Geometry: final body of the model. Coordinates: model frame, mm. Face numbers are marked on the shaded views. A direction names the side the tool comes from. Round coordinates to 2 decimals unless told otherwise and drop trailing zeros. Loops run counter-clockwise (first coordinate to the right, second up) from the corner with the lowest first, then second, coordinate; pieces in that order, holes last. Notation, with made-up numbers: M 38.5,79.5 L 50.5,79.5 A19 ccw 50.5,99.5 Z; hole C 50,26.25 d10. An arc over 180 degrees is marked long. Write each question's results on one line, items separated by ' | '.
```python
from build123d import *

# Parameters (mm, degrees)
F1_DEPTH  = 20
F2_R      = 2.65
F3_DEPTH  = 30.001
F4_R      = 2.75
F5_DEPTH  = 7
F6_W      = 30
F6_H      = 10
F7_DEPTH  = 10.1
F9_R      = 5
F8_W      = 30
F8_H      = 4.3
F10_DEPTH = 30.001
F11_R     = 5


with BuildPart() as f1:
    # F0 (on Front) → F1 (new body)
    with BuildSketch(Plane.XZ):
        Polygon((-0.255054, 4.627101), (-7.005054, 4.627101), (-7.005054, -20.372899), (-2.005054, -20.372899), (-2.005054, -0.472899), (1.994946, -0.472899), (1.994946, 7.327101), (13.994946, 7.327101), (13.994946, -0.472899), (17.994946, -0.472899), (17.994946, -20.372899), (22.994946, -20.372899), (22.994946, 4.627101), (16.244946, 4.627101), (16.244946, 9.627101), (-0.255054, 9.627101), align=None)
    extrude(amount=F1_DEPTH)

    # F2 (on face) → F3 (cut, through all)
    with BuildSketch(Plane(origin=(-7.005054, 0, 0), x_dir=(0, -1, 0), z_dir=(-1, 0, 0))):
        with Locations((10, -10.372899)):
            Circle(F2_R)
    extrude(amount=-F3_DEPTH, mode=Mode.SUBTRACT)

    # F4 (on face) → F5 (join)
    with BuildSketch(Plane.XY.offset(9.627101)):
        with Locations((7.994946, -13)):
            Circle(F4_R)
    extrude(amount=-F5_DEPTH)

    # F6 (on face) → F7 (cut, through all)
    with BuildSketch(Plane.XY.offset(9.627101)):
        with Locations((7.994946, -5)):
            Rectangle(F6_W, F6_H)
    extrude(amount=-F7_DEPTH, mode=Mode.SUBTRACT)

    # F9
    f9_edges = [f1.edges().sort_by_distance(p)[0] for p in [
        (20.494946, 0, -0.472899),
        (-4.505054, 0, -0.472899),
    ]]
    fillet(f9_edges, radius=F9_R)

    # F8 (on face) → F10 (cut, through all)
    with BuildSketch(Plane(origin=(0, 0, -20.372899), x_dir=(1, 0, 0), z_dir=(0, 0, -1))):
        with Locations((7.994946, 17.85)):
            Rectangle(F8_W, F8_H)
    extrude(amount=-F10_DEPTH, mode=Mode.SUBTRACT)

    # F11
    f11_edges = [f1.edges().sort_by_distance(p)[0] for p in [
        (20.494946, 0, -20.372899),
        (-4.505054, 0, -20.372899),
    ]]
    fillet(f11_edges, radius=F11_R)


solid = f1.part
```
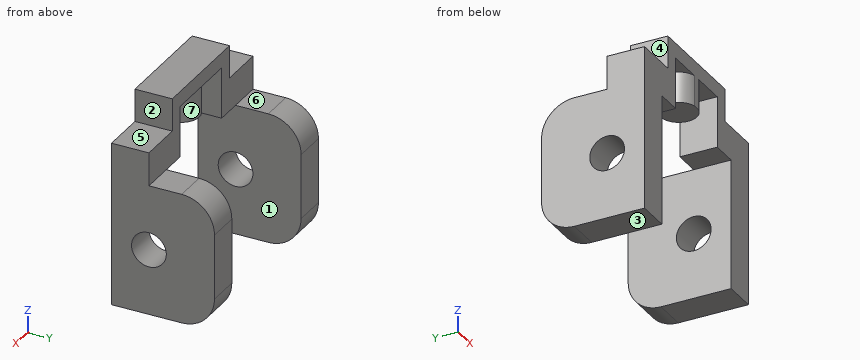
1. Section C-C (z = 5.5). Output: boundary loops of the cut face in (x, y), then the cut area to 3 significant figures.
Answer key:
outline: M -0.26,-15.7 L 1.99,-15.7 L 1.99,-10 L -0.26,-10 Z; M 7.47,-15.7 L 8.52,-15.7 A2.75 ccw long Z; M 13.99,-15.7 L 16.24,-15.7 L 16.24,-10 L 13.99,-10 Z | area: 49.4 mm²
2. Pin query (flat end, axial travel): P1, Ø6.5, axis at x = -4.5, y = -14, coming from the +Z side; P2, Ø2.5, axis at y = -11.5, z = 6, coming from the +X side; P3, Ø8, axis at x = 11, z = 6, coming from the +Y side. Return the tip coordinate at first contact, or that it passes through.
Answer key:
P1: stops at z = 4.63 | P2: stops at x = 16.24 | P3: stops at y = -10
3. Ray query, probe 1 along X at (y, z) = (-11.75, -7.5); probe 2 along X at (y, z) = (-11.25, 2.75); probe 3 along Z at (x, y) = (-1.25, -10.75). Return the intervals inside material, ascending.
Answer key:
probe 1: x = -7.01 to -2.01, 17.99 to 22.99 | probe 2: x = -7.01 to 1.99, 5.87 to 10.12, 13.99 to 22.99 | probe 3: z = -0.47 to 4.63
4. Draft query along X for the marked faces 1, 2 and 3. Return one class per face: pulls with the +X half, pulls with the -X half, needs draft (parallel to the pull), parting line crosses it, or undercut.
Answer key:
face 1: undercut | face 2: pulls with the +X half | face 3: needs draft
5. Section D-D (y = -13.75). Output: boundary loops of the cut face in (x, z).
Answer key:
outline: M -7.01,-20.37 L -2.01,-20.37 L -2.01,-0.47 L 1.99,-0.47 L 1.99,7.33 L 5.35,7.33 L 5.35,2.63 L 10.64,2.63 L 10.64,7.33 L 13.99,7.33 L 13.99,-0.47 L 17.99,-0.47 L 17.99,-20.37 L 22.99,-20.37 L 22.99,4.63 L 16.24,4.63 L 16.24,9.63 L -0.26,9.63 L -0.26,4.63 L -7.01,4.63 Z
6. Access query for the marked faces 4, 5, 6 and 7. Directions: +Z, -Z, +X, -X, +Y, -Y. A direction counts if a zero-diameter tool reaches every point of the face in a straight line with its end or side. Return the directions, or none.
Answer key:
face 4: +Z, -X, +Y, -Y | face 5: +Z, +X, +Y, -Y | face 6: +Z, +X, -X, +Y | face 7: -Z
7. Section B-B (y = -2.75). Output: boundary loops of the cut face in (x, z), then the cut area to 3 significant figures.
Answer key:
outline: M -7.01,-19.84 L -2.01,-19.84 L -2.01,-1.01 L -7.01,-1.01 Z; M 17.99,-19.84 L 22.99,-19.84 L 22.99,-1.01 L 17.99,-1.01 Z | area: 188 mm²
8. Section A-A (z = 0.25). Output: boundary loops of the cut face in (x, y), then the cut area to 3 significant figures.
Answer key:
outline: M -7.01,-15.7 L 1.99,-15.7 L 1.99,-10 L -7.01,-10 Z; M 13.99,-15.7 L 22.99,-15.7 L 22.99,-10 L 13.99,-10 Z | area: 103 mm²
